```python
from build123d import *

# Parameters (mm, degrees)
SKETCH1_W           = 120
SKETCH1_H           = 130
SKETCH1_R           = 1.4
SKETCH1_R_2         = 1.15
SKETCH1_R_3         = 2
SKETCH1_R_4         = 1.65
SKETCH1_W_2         = 14
SKETCH1_H_2         = 62
SKETCH1_W_3         = 2.5
SKETCH1_H_3         = 4
BOSS_EXTRUDE1_DEPTH = 3.175
FILLET1_R           = 10


with BuildPart() as part:
    # Sketch1 → Boss-Extrude1 (new body)
    with BuildSketch(Plane(origin=(0, 0, 0), x_dir=(1, 0, 0), z_dir=(0, 1, 0))):
        Rectangle(SKETCH1_W, SKETCH1_H)
        with Locations(Location((29, 14, 0), (0, 0, 270))):
            Circle(SKETCH1_R, mode=Mode.SUBTRACT)
        with Locations(Location((29, -9.05, 0), (0, 0, 270))):
            Circle(SKETCH1_R, mode=Mode.SUBTRACT)
        with Locations(Location((-29, -9.05, 0), (0, 0, 270))):
            Circle(SKETCH1_R, mode=Mode.SUBTRACT)
        with Locations(Location((-29, 14, 0), (0, 0, 270))):
            Circle(SKETCH1_R, mode=Mode.SUBTRACT)
        with Locations(Location((32.225, -15, 0), (0, 0, 270))):
            Circle(SKETCH1_R_2, mode=Mode.SUBTRACT)
        with Locations(Location((32.225, -33, 0), (0, 0, 270))):
            Circle(SKETCH1_R_2, mode=Mode.SUBTRACT)
        with Locations(Location((-32.225, -33, 0), (0, 0, 270))):
            Circle(SKETCH1_R_2, mode=Mode.SUBTRACT)
        with Locations(Location((-32.225, -15, 0), (0, 0, 270))):
            Circle(SKETCH1_R_2, mode=Mode.SUBTRACT)
        with Locations(Location((20, 52.5, 0), (0, 0, 270))):
            Circle(SKETCH1_R_3, mode=Mode.SUBTRACT)
        with Locations(Location((-20, 52.5, 0), (0, 0, 270))):
            Circle(SKETCH1_R_3, mode=Mode.SUBTRACT)
        with Locations(Location((53.217198973, -57.651965554, 0), (0, 0, 270))):
            Circle(SKETCH1_R_4, mode=Mode.SUBTRACT)
        with Locations(Location((53.217198973, 57.651965554, 0), (0, 0, 270))):
            Circle(SKETCH1_R_4, mode=Mode.SUBTRACT)
        with Locations(Location((-53.217198973, -57.651965554, 0), (0, 0, 270))):
            Circle(SKETCH1_R_4, mode=Mode.SUBTRACT)
        with Locations(Location((-53.217198973, 57.651965554, 0), (0, 0, 270))):
            Circle(SKETCH1_R_4, mode=Mode.SUBTRACT)
        with Locations(Location((-15, -45, 0), (0, 0, 270))):
            Circle(SKETCH1_R_4, mode=Mode.SUBTRACT)
        with Locations(Location((15, -45, 0), (0, 0, 270))):
            Circle(SKETCH1_R_4, mode=Mode.SUBTRACT)
        with Locations((-43.475, -24)):
            Rectangle(SKETCH1_W_2, SKETCH1_H_2, mode=Mode.SUBTRACT)
        with Locations((43.475, -24)):
            Rectangle(SKETCH1_W_2, SKETCH1_H_2, mode=Mode.SUBTRACT)
        with Locations((45.25, 33)):
            Rectangle(SKETCH1_W_3, SKETCH1_H_3, mode=Mode.SUBTRACT)
        with Locations((-45.25, 33)):
            Rectangle(SKETCH1_W_3, SKETCH1_H_3, mode=Mode.SUBTRACT)
    extrude(amount=BOSS_EXTRUDE1_DEPTH)

    # Fillet1
    fillet1_edges = [part.edges().sort_by_distance(p)[0] for p in [
        (60, 1.5875, 65),
        (-60, 1.5875, 65),
        (-60, 1.5875, -65),
        (60, 1.5875, -65),
    ]]
    fillet(fillet1_edges, radius=FILLET1_R)


solid = part.part
```
Geometry: final body of the model. Coordinates: model frame, mm. A direction names the side the tool comes from. Coordinates: 2 decimals unless noted, no trailing zeros. Write each loop counter-clockwise with the first axis right and the second up, starting at its lowest first coordinate (ties: lowest second). Pieces come first, ordered by that corner, then holes. Notation, with made-up numbers: M -13,53.5 L 2,53.5 A7 cw 2,66.5 Z; hole C 17,28 d3. An arc over 180 degrees is marked long. Use CSV: the item, a comma, the result in double quotes. Start each with the question number.
1. Cut plane B-B on z = 4.5. Return the cut outline in (x, y) (3 decimals), plus the area to 3 significant figures.
2. Reachability of faces 1 (the face through (-57.15, 1.61, -61.99)), 2 (the face through (43, 2, 55)) from +Z, -Z, +X, -X, +Y, -Y: full face, straight path, thin tool, end or side. Return the list, or none.
3. Cut plane C-C on x = 20. Return the cut outline in (y, z) (3 decimals), plus the area to 3 significant figures.
4. Ray query, probe 1 along X at (y, z) = (1.25, 33) (3 decimals); probe 2 along X at (y, z) = (2.2, -52.5); probe 3 along X at (y, z) = (0.55, 41) (3 decimals). Return the intervals inside material, ascending.
5. Mould query, pull axis Z, two halves, no side actions, for faces 3 (the face through (51.753, 1.565, -56.891)), 4 (the face through (60, 2, 1)), 5 (the face through (-36.475, 2, 24)), 6 (the face through (-57.15, 1.61, 61.99)). Classes: pulls with the +Z half, pulls with the -Z half, needs draft (parallel to the pull), parting line crosses it, or undercut.
6. Cut plane A-A on x = -15. Return the cut outline in (y, z) (3 decimals).
7. Cut plane D-D on y = 0.7. Count the separate pieces of the cut face and the enclosed holes in it, plus the area to 3 significant figures.
Entries:
1,outline,"M -60,0 L -50.475,0 L -50.475,3.175 L -60,3.175 Z; M -36.475,0 L 36.475,0 L 36.475,3.175 L -36.475,3.175 Z; M 50.475,0 L 60,0 L 60,3.175 L 50.475,3.175 Z"
1,area,"292 mm²"
2,face 1,"-Z, -X, +Y, -Y"
2,face 2,"+Y, -Y"
3,outline,"M 0,-65 L 3.175,-65 L 3.175,-54.5 L 0,-54.5 Z; M 0,-50.5 L 3.175,-50.5 L 3.175,65 L 0,65 Z"
3,area,"400 mm²"
4,probe 1,"-60 to -50.475, -36.475 to -33.375, -31.075 to 31.075, 33.375 to 36.475, 50.475 to 60"
4,probe 2,"-60 to -22, -18 to 18, 22 to 60"
4,probe 3,"-60 to -50.475, -36.475 to 36.475, 50.475 to 60"
5,face 3,"undercut"
5,face 4,"needs draft"
5,face 5,"undercut"
5,face 6,"pulls with the +Z half"
6,outline,"M 0,-65 L 3.175,-65 L 3.175,43.35 L 0,43.35 Z; M 0,46.65 L 3.175,46.65 L 3.175,65 L 0,65 Z"
7,separate pieces,"1"
7,enclosed holes,"20"
7,area,"13,600 mm²"
